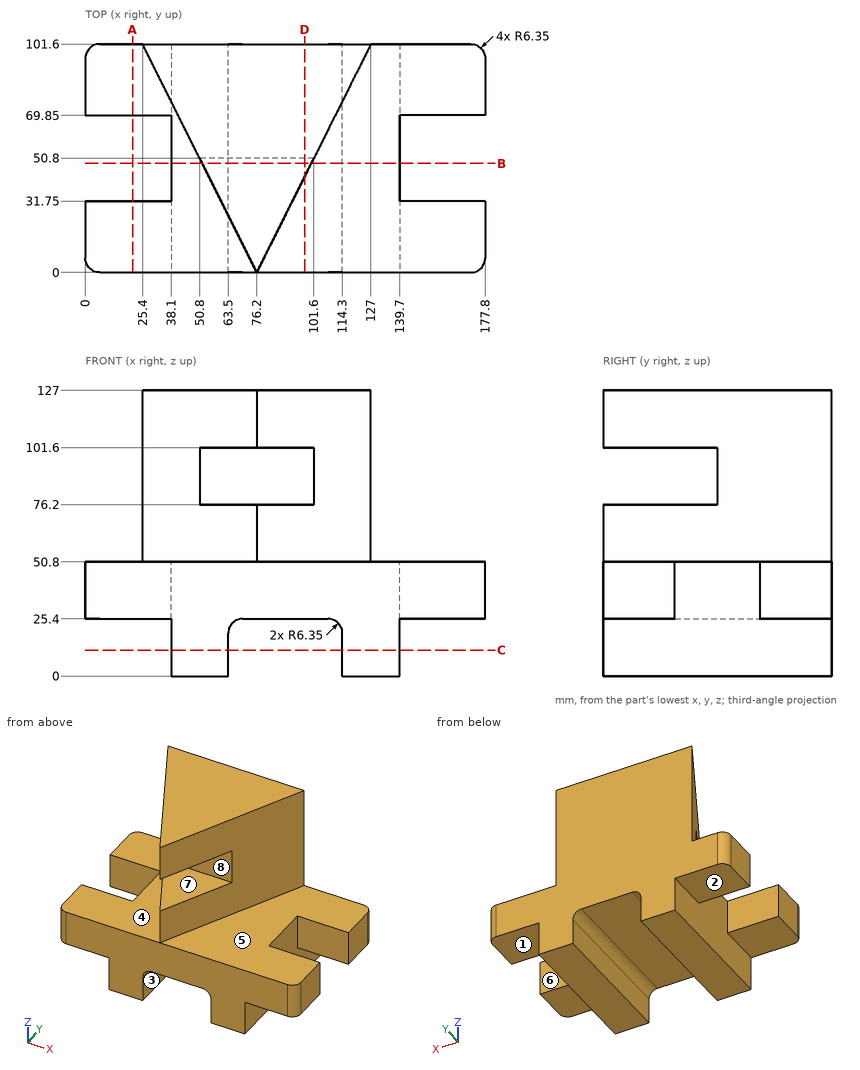
Part print with two shaded views. Sizes in mm from the minimum x, y, z corner. A direction names the side the tool comes from. Round coordinates to 2 decimals unless told otherwise and drop trailing zeros. Write each loop counter-clockwise with the first axis right and the second up, starting at its lowest first coordinate (ties: lowest second). Pieces come first, ordered by that corner, then holes. Notation, with made-up numbers: (28.5, -18.5) -> (37.5, -18.5) arc R18 cw to (37.5, -7.5) -> close; hole circle Ø2 at (33.25, 9). An arc over 180 degrees is marked (long way). Put each result on its own line as item: value.
Item 1: Tool access for the marked faces 1, 2, 3 and 4: list every direction of +Z, -Z, +X, -X, +Y, -Y with a clear straight run to the whole face (end or side of a thin tool).
Here are the results:
face 1: -Z, +X, +Y, -Y
face 2: -Z, -X, +Y, -Y
face 3: -Z, +Y, -Y
face 4: +Z, -X, -Y
Item 2: Slice it at D-D, the plane x = 97.5. Give the cut face in (y, z), plus the area to 3 significant figures.
Here are the results:
outline: (0, 25.4) -> (101.6, 25.4) -> (101.6, 127) -> (42.6, 127) -> (42.6, 101.6) -> (50.8, 101.6) -> (50.8, 76.2) -> (42.6, 76.2) -> (42.6, 50.8) -> (0, 50.8) -> close
area: 6,870 mm^2
Item 3: Wall check: probe 1 along Y at (x, z) = (142, 49); probe 2 along Z at (x, y) = (73.5, 32); probe 3 along Z at (x, y) = (19.5, 23). Give the ranges that are in metal, low to high. Write a range as from..to.
Here are the results:
probe 1: y = 0..31.75, 69.85..101.6
probe 2: z = 25.4..76.2, 101.6..127
probe 3: z = 25.4..50.8
Item 4: Slice it at B-B, the plane y = 48.5. Give the cut face in (x, z).
Here are the results:
outline: (38.1, 0) -> (63.5, 0) -> (63.5, 19.05) arc R6.35 cw to (69.85, 25.4) -> (107.95, 25.4) arc R6.35 cw to (114.3, 19.05) -> (114.3, 0) -> (139.7, 0) -> (139.7, 50.8) -> (100.45, 50.8) -> (100.45, 76.2) -> (51.95, 76.2) -> (51.95, 50.8) -> (38.1, 50.8) -> close; (51.95, 101.6) -> (100.45, 101.6) -> (100.45, 127) -> (51.95, 127) -> close
Item 5: Two-plate mould, pull along Z, no slides. Class the marked faces 5, 6, 7 and 8: pulls with the +Z half, pulls with the -Z half, needs draft (parallel to the pull), parting line crosses it, or undercut.
Here are the results:
face 5: pulls with the +Z half
face 6: needs draft
face 7: undercut
face 8: undercut
Item 6: Slice it at C-C, the plane z = 11.5. Give the cut face in (x, y).
Here are the results:
outline: (38.1, 0) -> (63.5, 0) -> (63.5, 101.6) -> (38.1, 101.6) -> close; (114.3, 0) -> (139.7, 0) -> (139.7, 101.6) -> (114.3, 101.6) -> close
Item 7: Slice it at A-A, the plane x = 21. Give the cut face in (y, z), plus the area to 3 significant figures.
Here are the results:
outline: (0, 25.4) -> (31.75, 25.4) -> (31.75, 50.8) -> (0, 50.8) -> close; (69.85, 25.4) -> (101.6, 25.4) -> (101.6, 50.8) -> (69.85, 50.8) -> close
area: 1,610 mm^2
Item 8: Flat gauge pins, fed straight in: P1, Ø9.5, axis at x = 157, y = 22, coming from the -Z side; P2, Ø15, axis at y = 48.5, z = 5.5, coming from the -X side; P3, Ø8, axis at y = 32, z = 68, coming from the +X side. Where does each tip first touch, or does it go through?
Here are the results:
P1: stops at z = 25.4
P2: stops at x = 38.1
P3: stops at x = 94.2
